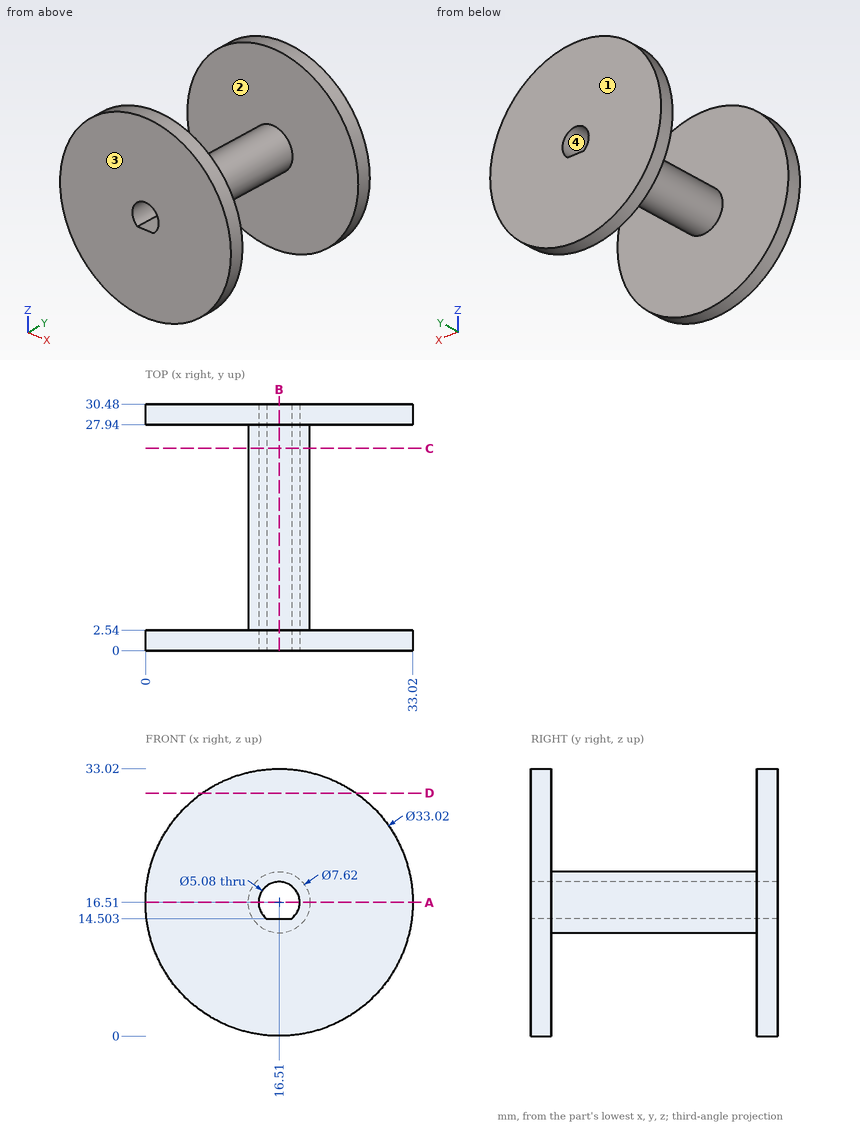
Could you check a few things on this drawing? It's one solid part, dimensions in mm from its lowest x, y, z. Coordinates: 2 decimals unless noted, no trailing zeros. Order: outer loops, then holes, each group sorted by start corner. A loop starts at its lowest first (then second) coordinate and runs counter-clockwise, first axis right, second up.
1) Imagine slicing it at D-D on z = 30. List the corners of the cut face in (x, y) for me.
2) I need wall thicknesses on line 1 (X direction, y = 20, z = 16.51); line 2 (Y direction, x = 22.5, z = 16); line 3 (Z direction, x = 16.5, y = 29.5). Which ranges of each line are inside material? Lowest first, please.
3) Will these pins go through, and if not, where does the flat tip stop? pin 1 (6 mm diameter, centred on y = 25.5, z = 23, fed in from -X); pin 2 (2.5 mm diameter, centred on x = 16, y = 7.5, fed in from +Z); pin 3 (10 mm diameter, centred on x = 20.5, y = 6, fed in from +Z).
4) We'd pull the mould along Y, two halves only. Please class the marked faces 1, 2, 3 and 4: +Y half, -Y half, draft (parallel to the pull), parting line (faces both ways), or undercut.
5) Imagine slicing it at A-A on z = 16.51. List the corners of the cut face in (x, y) for me.
6) Imagine slicing it at B-B on x = 16.51. List the corners of the cut face in (y, z) for me.
7) Imagine slicing it at C-C on y = 25. List the corners of the cut face in (x, z) for me.
Response values:
1. outline: (6.99, 0) - (26.03, 0) - (26.03, 2.54) - (6.99, 2.54) - close; (6.99, 27.94) - (26.03, 27.94) - (26.03, 30.48) - (6.99, 30.48) - close
2. line 1: x = 12.7 to 13.97, 19.05 to 20.32
2. line 2: y = 0 to 2.54, 27.94 to 30.48
2. line 3: z = 0 to 14.5, 19.05 to 33.02
3. pin 1: stops at x = 0.7
3. pin 2: stops at z = 20.32
3. pin 3: stops at z = 33.02
4. face 1: +Y half
4. face 2: undercut
4. face 3: -Y half
4. face 4: draft
5. outline: (0, 0) - (13.97, 0) - (13.97, 30.48) - (0, 30.48) - (0, 27.94) - (12.7, 27.94) - (12.7, 2.54) - (0, 2.54) - close; (19.05, 0) - (33.02, 0) - (33.02, 2.54) - (20.32, 2.54) - (20.32, 27.94) - (33.02, 27.94) - (33.02, 30.48) - (19.05, 30.48) - close
6. outline: (0, 0) - (2.54, 0) - (2.54, 12.7) - (27.94, 12.7) - (27.94, 0) - (30.48, 0) - (30.48, 14.5) - (0, 14.5) - close; (0, 19.05) - (30.48, 19.05) - (30.48, 33.02) - (27.94, 33.02) - (27.94, 20.32) - (2.54, 20.32) - (2.54, 33.02) - (0, 33.02) - close
7. outline: circle Ø7.62 at (16.51, 16.51); hole (14.95, 14.5) - (18.07, 14.5) arc R2.54 ccw (long way) to start
